Work out the finished part from the listing and answer in its coordinate system (mm). Round coordinates to 2 decimals unless told otherwise and drop trailing zeros. Write each loop counter-clockwise with the first axis right and the second up, starting at its lowest first coordinate (ties: lowest second). Pieces come first, ordered by that corner, then holes. Notation, with made-up numbers: (8, 61.5) - (15, 61.5) arc R12 ccw to (15, 75.5) - close; hole circle Ø8 at (-40, 87). An arc over 180 degrees is marked (long way). Answer as a JSON object with one key per item and string values.
```python
from build123d import *
from OCP.BRepFilletAPI import BRepFilletAPI_MakeChamfer

# Parameters (mm, degrees)
BOSS_EXTRU_1_DEPTH = 10
CHANFREIN1_SIZE    = 60
CHANFREIN1_SIZE2   = 34.641016151


with BuildPart() as part:
    # Esquisse1 → Boss.-Extru.1 (new body)
    with BuildSketch(Plane.XY):
        Polygon((0, 0), (1080, 0), (1080, 90), (1040, 90), (1040, 10), (1000, 10), (1000, 90), (920, 90), (920, 10), (880, 10), (880, 90), (650, 90), (650, 10), (610, 10), (610, 90), (490, 90), (490, 10), (450, 10), (450, 90), (200, 90), (200, 10), (160, 10), (160, 90), (80, 90), (80, 10), (40, 10), (40, 90), (0, 90), align=None)
    extrude(amount=BOSS_EXTRU_1_DEPTH)

    # Chanfrein1: one chamfer whose edges measure the first distance from different faces: ONE call of the kernel's chamfer builder (chamfer() names one face for all edges)
    chanfrein1_edges_1 = [part.edges().sort_by_distance(p)[0] for p in [
        (0, 90, 5),
    ]]
    chanfrein1_side_1 = [part.faces().sort_by_distance(p)[0] for p in [
        (0, 45, 5),
    ]]
    chanfrein1_edges_2 = [part.edges().sort_by_distance(p)[0] for p in [
        (1080, 90, 5),
    ]]
    chanfrein1_side_2 = [part.faces().sort_by_distance(p)[0] for p in [
        (1080, 45, 5),
    ]]
    chanfrein1 = BRepFilletAPI_MakeChamfer(part.part.solid().wrapped)
    for e in chanfrein1_edges_1:
        chanfrein1.Add(CHANFREIN1_SIZE, CHANFREIN1_SIZE2, e.wrapped, chanfrein1_side_1[0].wrapped)  # the first distance lies on this face
    for e in chanfrein1_edges_2:
        chanfrein1.Add(CHANFREIN1_SIZE, CHANFREIN1_SIZE2, e.wrapped, chanfrein1_side_2[0].wrapped)  # the first distance lies on this face
    add(Compound.cast(chanfrein1.Shape()), mode=Mode.REPLACE)


solid = part.part
```
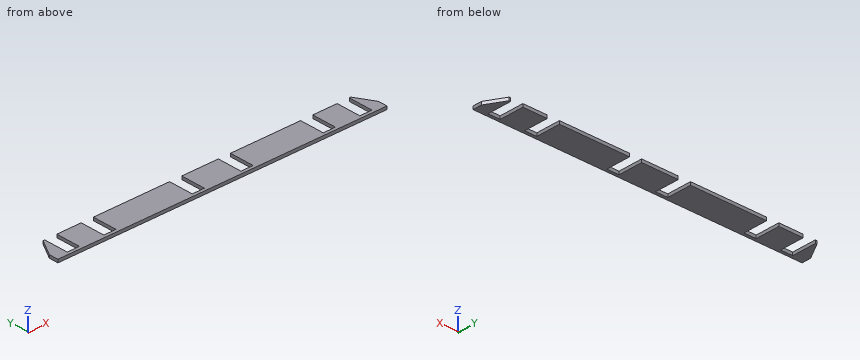
Item 1: Consider line 1 along Y through (x, z) = (479, 1). Determine where the line is inside the solid, lowest interval first.
Results found:
{"line 1": "0 to 10"}
Item 2: Each of these flat-tipped pins is pushed along its axis until it touches: P1, Ø1.5, axis at x = 891, z = 8, coming from the +Y side; P2, Ø3, axis at y = 61, z = 3, coming from the -X side; P3, Ø5, axis at y = 61, z = 4.5, coming from the -X side. Where does it stop, or does it pass through?
Results found:
{"P1": "y = 10", "P2": "x = 17.03", "P3": "x = 16.45"}
Item 3: A cutting plane is placed at A-A (y = 78.5). Write down the section's boundary in (x, z).
Results found:
{"outline": "(28, 0) - (40, 0) - (40, 10) - (28, 10) - close; (80, 0) - (160, 0) - (160, 10) - (80, 10) - close; (200, 0) - (450, 0) - (450, 10) - (200, 10) - close; (490, 0) - (610, 0) - (610, 10) - (490, 10) - close; (650, 0) - (880, 0) - (880, 10) - (650, 10) - close; (920, 0) - (1000, 0) - (1000, 10) - (920, 10) - close; (1040, 0) - (1052, 0) - (1052, 10) - (1040, 10) - close"}
